The figure shows three views and two pictorial views of one solid part (mm, origin at its lowest corner). Answer the questions. Round coordinates to 2 decimals unless told otherwise and drop trailing zeros. Order: outer loops, then holes, each group sorted by start corner. A loop starts at its lowest first (then second) coordinate and runs counter-clockwise, first axis right, second up. Notation, with made-up numbers: (87, 18) -> (136, 18) arc R25 ccw to (136, 47) -> close; hole circle Ø10 at (-28.75, -36.75). An arc over 180 degrees is marked (long way). One line per item, written item: value. Start each with the question number.
1. Section A-A (x = 22) is taken. Give the vertices of the cut face in (y, z).
2. Section B-B (y = 1.75) is taken. Give the vertices of the cut face in (x, z), then the cut area to 3 significant figures.
3. Flat-ended cylindrical pins translate along their axes: pin 1 Ø1.5 at (x, y) = (37, 1) entering from -Z; pin 2 Ø1.5 at (y, z) = (1.5, 2) entering from +X; pin 3 Ø3 at (x, z) = (54.5, 6.5) entering from -Y. Find the tip coordinate at first contact, or state that the pin passes through.
4. Section D-D (x = 12) is taken. Give the vertices of the cut face in (y, z), then the cut area to 3 significant figures.
5. Consider line 1 (X direction, y = 2.65, z = 26.5); line 2 (X direction, y = 2, z = 23); line 3 (Z direction, x = 48, y = 1.75). Determine where each line is inside the solid, lowest interval first.
6. Section C-C (z = 25) is taken. Give the vertices of the cut face in (x, y), then the cut area to 3 significant figures.
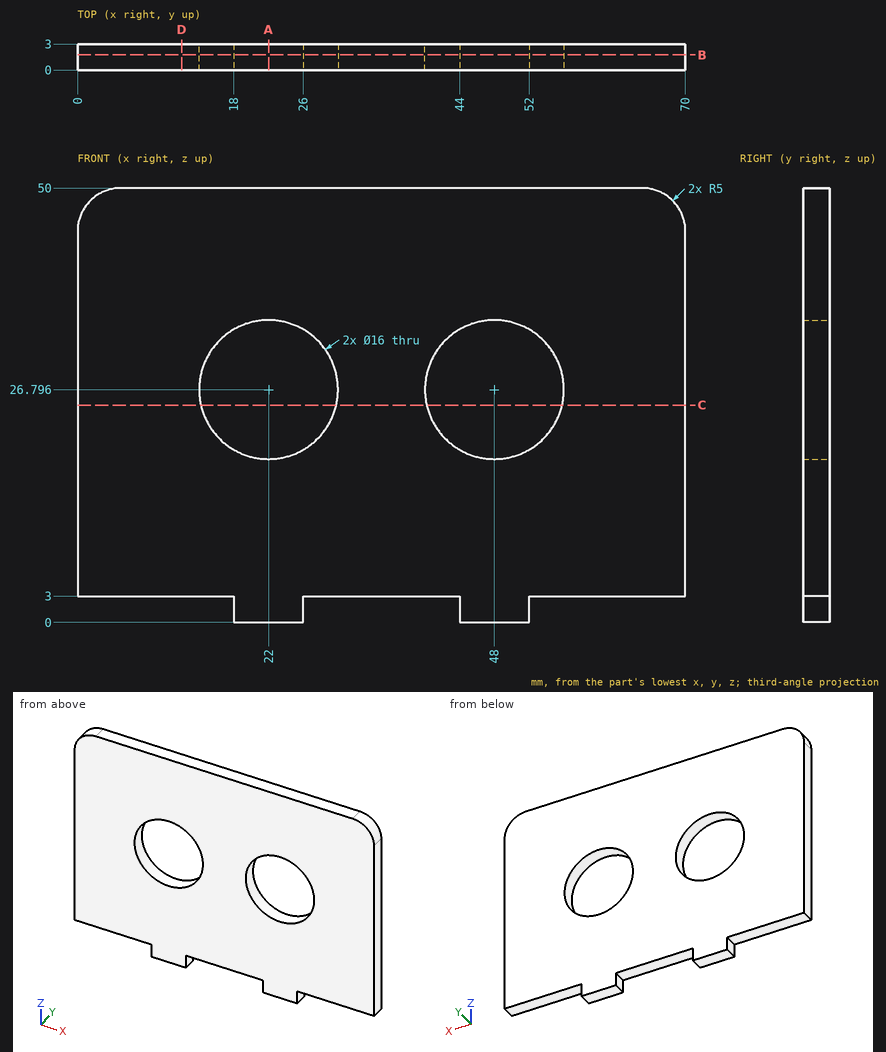
Answer:
1. outline: (0, 0) -> (3, 0) -> (3, 18.8) -> (0, 18.8) -> close; (0, 34.8) -> (3, 34.8) -> (3, 50) -> (0, 50) -> close
2. outline: (0, 3) -> (18, 3) -> (18, 0) -> (26, 0) -> (26, 3) -> (44, 3) -> (44, 0) -> (52, 0) -> (52, 3) -> (70, 3) -> (70, 45) arc R5 ccw to (65, 50) -> (5, 50) arc R5 ccw to (0, 45) -> close; hole circle Ø16 at (22, 26.8); hole circle Ø16 at (48, 26.8)
2. area: 2,930 mm^2
3. pin 1: z = 3
3. pin 2: x = 52
3. pin 3: y = 0
4. outline: (0, 3) -> (3, 3) -> (3, 50) -> (0, 50) -> close
4. area: 141 mm^2
5. line 1: 0 to 14.01, 29.99 to 40.01, 55.99 to 70
5. line 2: 0 to 14.96, 29.04 to 40.96, 55.04 to 70
5. line 3: 0 to 18.8, 34.8 to 50
6. outline: (0, 0) -> (14.2, 0) -> (14.2, 3) -> (0, 3) -> close; (29.8, 0) -> (40.2, 0) -> (40.2, 3) -> (29.8, 3) -> close; (55.8, 0) -> (70, 0) -> (70, 3) -> (55.8, 3) -> close
6. area: 116 mm^2
